Work out the finished part from the listing and answer in its coordinate system (mm). Face numbers are marked on the shaded views. A direction names the side the tool comes from. Coordinates: 2 decimals unless noted, no trailing zeros. Write each loop counter-clockwise with the first axis right and the second up, starting at its lowest first coordinate (ties: lowest second). Pieces come first, ordered by that corner, then holes. Notation, with made-up numbers: (-29, 41.5) - (4, 41.5) arc R24 ccw to (4, 59.5) - close; hole circle Ø8 at (59.5, 69). An arc over 180 degrees is marked (long way). Use a Markdown table: item, result. Add a question column.
(1) The part is cut by section A-A, the plane y = 1.5. Give the vertices of the cut face in (x, z) (3 decimals), then the cut area to 3 significant figures.
(2) The part is cut by section C-C, the plane x = 19. Give the vertices of the cut face in (y, z).
(3) Given pin 1 Ø1.5 at (y, z) = (5, -2) entering from +X (3 decimals); pin 2 Ø0.7 at (x, y) = (9, 6) entering from -Z; pin 3 Ø0.7 at (x, y) = (9, 6.5) entering from +Z, each flat-ended and moving along its own axis, determine where each tip first touches the part or whether it passes through.
(4) For a pull along X with two mould halves and no side action, classify the marked faces 1, 2, 3 and 4 as released by +X, released by -X, zero draft, split by the parting line, or undercut.
(5) A tool of negligible diameter and unlimited length cuts with its end or side. For the marked faces 5, 6 and 7, from which of +Z, -Z, +X, -X, +Y, -Y can it reach the whole face along a straight path? Write none if from no direction.
(6) The part is cut by section B-B, the plane x = 3.5. Give the vertices of the cut face in (y, z) (1 decimal).
(7) Find the intervals of material crossed by line 1 (X direction, y = -1.3, z = 0); line 2 (X direction, y = 4.25, z = 1.5) (3 decimals); line 3 (X direction, y = -0.65, z = 0), in increasing order. Write a range as from..to.
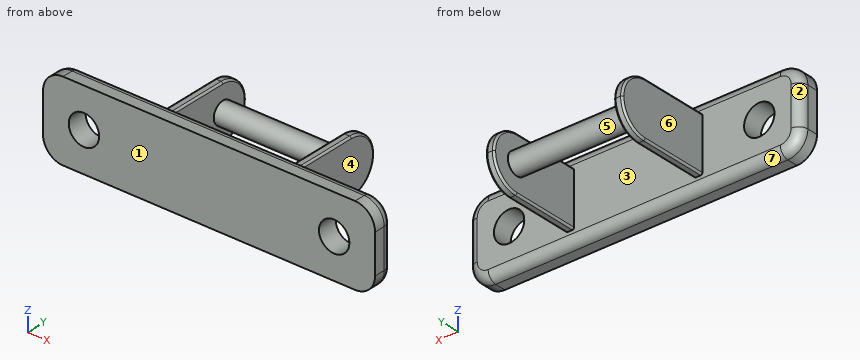
from build123d import *

# Parameters (mm, degrees)
SKETCH1_W           = 46.355
SKETCH1_H           = 11.049
SKETCH1_R           = 2.1209
BOSS_EXTRUDE1_DEPTH = 2.794
SKETCH2_W           = 1.143
SKETCH2_H           = 7.62
BOSS_EXTRUDE2_DEPTH = 13.335
FILLET1_R           = 3.81
SKETCH3_R           = 1.524
BOSS_EXTRUDE3_DEPTH = 16.764
FILLET2_R           = 2.794
FILLET3_R           = 1.27
FILLET4_R           = 0.254


with BuildPart() as part:
    # Sketch1 → Boss-Extrude1 (new body)
    with BuildSketch(Plane(origin=(0, 0, 0), x_dir=(1, 0, 0), z_dir=(0, 1, 0))):
        Rectangle(SKETCH1_W, SKETCH1_H)
        with Locations(Location((-17.4625, 0, 0), (0, 0, 270))):
            Circle(SKETCH1_R, mode=Mode.SUBTRACT)
        with Locations(Location((17.4625, 0, 0), (0, 0, 90))):
            Circle(SKETCH1_R, mode=Mode.SUBTRACT)
    extrude(amount=-BOSS_EXTRUDE1_DEPTH)

    # Sketch2 → Boss-Extrude2 (add)
    with BuildSketch(Plane(origin=(0, 0, 0), x_dir=(1, 0, 0), z_dir=(0, 1, 0))):
        with Locations((8.9535, 0)):
            Rectangle(SKETCH2_W, SKETCH2_H)
        with Locations((-8.9535, 0)):
            Rectangle(SKETCH2_W, SKETCH2_H)
    extrude(amount=BOSS_EXTRUDE2_DEPTH)

    # Fillet1
    fillet1_edges = [part.edges().sort_by_distance(p)[0] for p in [
        (-8.9535, 13.335, -3.81),
        (-8.9535, 13.335, 3.81),
        (8.9535, 13.335, -3.81),
        (8.9535, 13.335, 3.81),
    ]]
    fillet(fillet1_edges, radius=FILLET1_R - 0.0001)  # a hair under: the kernel refuses the full size

    # Sketch3 → Boss-Extrude3 (add)
    with BuildSketch(Plane(origin=(-8.382, 0, 0), x_dir=(0, 0, -1), z_dir=(1, 0, 0))):
        with Locations(Location((0, 9.525, 0), (0, 0, 180))):
            Circle(SKETCH3_R)
    extrude(amount=BOSS_EXTRUDE3_DEPTH)

    # Fillet2
    fillet2_edges = [part.edges().sort_by_distance(p)[0] for p in [
        (-23.1775, -1.397, -5.5245),
        (23.1775, -1.397, -5.5245),
        (23.1775, -1.397, 5.5245),
        (-23.1775, -1.397, 5.5245),
    ]]
    fillet(fillet2_edges, radius=FILLET2_R)

    # Fillet3
    fillet3_edges = [part.edges().sort_by_distance(p)[0] for p in [
        (0, 0, 5.5245),
        (-23.1775, 0, 0),
        (23.1775, 0, 0),
        (0, 0, -5.5245),
        (-22.359156347, 0, 4.706156347),
        (-22.359156347, 0, -4.706156347),
        (22.359156347, 0, -4.706156347),
        (22.359156347, 0, 4.706156347),
    ]]
    fillet(fillet3_edges, radius=FILLET3_R)

    # Fillet4
    fillet4_edges = [part.edges().sort_by_distance(p)[0] for p in [
        (-9.525, 4.76255, 3.81),
        (-9.525, 4.76255, -3.81),
        (-9.525, 12.219106126, 2.694106126),
        (-9.525, 12.219106126, -2.694106126),
        (-8.382, 4.76255, -3.81),
        (-8.382, 4.76255, 3.81),
        (-8.382, 12.219106126, 2.694106126),
        (-8.382, 12.219106126, -2.694106126),
        (8.382, 4.76255, 3.81),
        (8.382, 4.76255, -3.81),
        (8.382, 12.219106126, 2.694106126),
        (8.382, 12.219106126, -2.694106126),
        (9.525, 4.76255, -3.81),
        (9.525, 4.76255, 3.81),
        (9.525, 12.219106126, 2.694106126),
        (9.525, 12.219106126, -2.694106126),
    ]]
    fillet(fillet4_edges, radius=FILLET4_R)


solid = part.part
Model answer:
| question | item | result |
|---|---|---|
| 1 | outline | (-9.525, -3.556) arc R0.254 ccw to (-9.271, -3.81) - (-8.636, -3.81) arc R0.254 ccw to (-8.382, -3.556) - (-8.382, 3.556) arc R0.254 ccw to (-8.636, 3.81) - (-9.271, 3.81) arc R0.254 ccw to (-9.525, 3.556) - close; (8.382, -3.556) arc R0.254 ccw to (8.636, -3.81) - (9.271, -3.81) arc R0.254 ccw to (9.525, -3.556) - (9.525, 3.556) arc R0.254 ccw to (9.271, 3.81) - (8.636, 3.81) arc R0.254 ccw to (8.382, 3.556) - close |
| 1 | area | 17.3 mm^2 |
| 2 | outline | (-2.79, -5.52) - (-1.27, -5.52) arc R1.27 ccw to (0, -4.25) - (0, -1.46) - (-2.79, -1.46) - close; (-2.79, 1.46) - (0, 1.46) - (0, 4.25) arc R1.27 ccw to (-1.27, 5.52) - (-2.79, 5.52) - close |
| 3 | pin 1 | x = 9.525 |
| 3 | pin 2 | z = -3.81 |
| 3 | pin 3 | z = 3.81 |
| 4 | face 1 | zero draft |
| 4 | face 2 | released by -X |
| 4 | face 3 | undercut |
| 4 | face 4 | released by +X |
| 5 | face 5 | none |
| 5 | face 6 | +Z, -Z, -X, +Y |
| 5 | face 7 | -Z, +X, -X, +Y |
| 6 | outline | (-2.8, -5.5) - (-1.3, -5.5) arc R1.3 ccw to (0, -4.3) - (0, 4.3) arc R1.3 ccw to (-1.3, 5.5) - (-2.8, 5.5) - close; circle Ø3 at (9.5, 0) |
| 7 | line 1 | -23.18..-19.58, -15.34..15.34, 19.58..23.18 |
| 7 | line 2 | -9.525..-8.382, 8.382..9.525 |
| 7 | line 3 | -23.02..-19.58, -15.34..15.34, 19.58..23.02 |
